Input: dimensioned drawing with shaded views. Units: mm. Origin: part minimum x, y, z. A direction names the side the tool comes from. Round coordinates to 2 decimals unless told otherwise and drop trailing zeros. Write each loop counter-clockwise with the first axis right and the second up, starting at its lowest first coordinate (ties: lowest second). Pieces come first, ordered by that corner, then holes. Notation, with made-up numbers: (72.25, 53) - (125.25, 53) arc R21 ccw to (125.25, 63) - close; hole circle Ø1 at (5, -8). An arc over 180 degrees is marked (long way). Use one line per item in the form item = value.
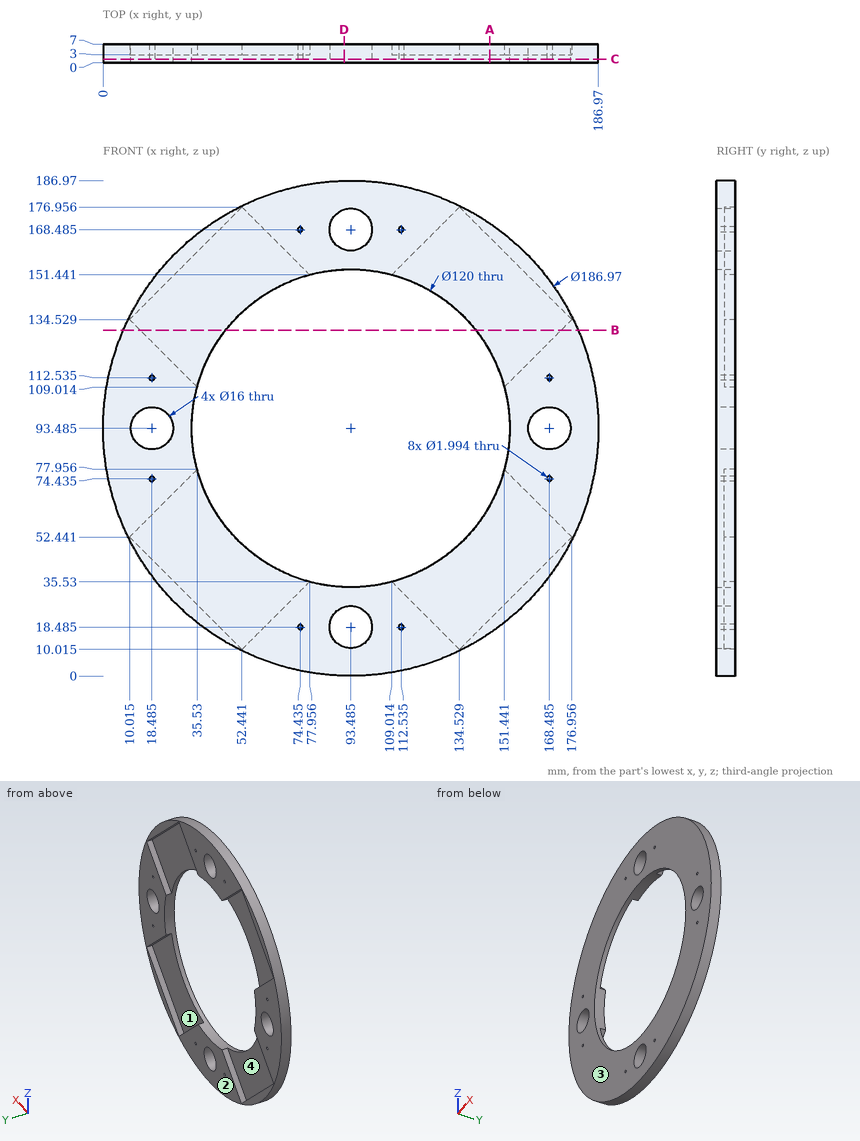
(1) First-contact query: pin 1 Ø21 at (x, z) = (93.49, 168.49) entering from +Y; pin 2 Ø8 at (x, z) = (143.5, 136) entering from +Y; pin 3 Ø3 at (y, z) = (3.5, 43) entering from +X; pin 4 Ø3 at (y, z) = (5, 87.5) entering from +X. Flat tips, straight axial feed; report the tip coordinate or a pass-through.
Derived:
pin_1 = 7
pin_2 = 3
pin_3 = 173.11
pin_4 = 186.86
(2) Cut plane C-C on y = 1.25. Count the separate pieces of the cut face and the enclosed holes in it, then the cut area to 3 significant figures.
Derived:
separate_pieces = 1
enclosed_holes = 13
area = 15,300 mm^2
(3) Cut plane B-B on z = 130.5. Output: boundary loops of the cut face in (x, y), then the cut area to 3 significant figures.
Derived:
outline = (7.64, 0) - (46.26, 0) - (46.26, 3) - (14.04, 3) - (14.04, 7) - (7.64, 7) - close; (140.71, 0) - (179.33, 0) - (179.33, 7) - (172.93, 7) - (172.93, 3) - (140.71, 3) - close
area = 283 mm^2
(4) Cut plane A-A on x = 146. Output: boundary loops of the cut face in (y, z) (1 decimal).
Derived:
outline = (0, 16.1) - (7, 16.1) - (7, 21.5) - (3, 21.5) - (3, 64.5) - (0, 64.5) - close; (0, 122.5) - (3, 122.5) - (3, 165.5) - (7, 165.5) - (7, 170.8) - (0, 170.8) - close
(5) Access query for the marked faces 3 and 4. Directions: +Z, -Z, +X, -X, +Y, -Y. A direction counts if a zero-diameter tool reaches every point of the face in a straight line with its end or side. Return the directions, or none.
Derived:
face_3 = +Z, -Z, +X, -X, -Y
face_4 = +Y
(6) Cut plane D-D on x = 91. Output: boundary loops of the cut face in (y, z), then the cut area to 3 significant figures.
Derived:
outline = (0, 0.03) - (7, 0.03) - (7, 10.88) - (0, 10.88) - close; (0, 26.09) - (7, 26.09) - (7, 33.54) - (0, 33.54) - close; (0, 153.43) - (7, 153.43) - (7, 160.88) - (0, 160.88) - close; (0, 176.09) - (7, 176.09) - (7, 186.94) - (0, 186.94) - close
area = 256 mm^2
(7) Draft query along X for the marked faces 1 and 2. Return one class per face: released by +X, released by -X, zero draft, split by the parting line, or undercut.
Derived:
face_1 = undercut
face_2 = zero draft
(8) Material intervals for L1, parallel to Z at x = 170, y = 3.75 (1 decimal); L2, parallel to X at y = 1, z = 18 (1 decimal); L3, parallel to X at y = 4.75, z = 169 (1 decimal), sorted ascending.
Derived:
L1 = 39.8 to 45.5, 59.4 to 85.6, 101.3 to 127.6, 141.5 to 147.2
L2 = 38.3 to 73.6, 75.3 to 85.5, 101.5 to 111.7, 113.4 to 148.6
L3 = 38.4 to 44.5, 60.4 to 73.6, 75.3 to 85.5, 101.5 to 111.7, 113.4 to 126.6, 142.5 to 148.6
